from build123d import *

# Parameters (mm, degrees)
BOSS_EXTRUDE1_DEPTH      = 10.5
BOSS_EXTRUDE1_DEPTH_BACK = 10.5
SKETCH1_R                = 26.5
SKETCH1_R_2              = 7.5
BOSS_EXTRUDE2_DEPTH      = 8
BOSS_EXTRUDE2_DEPTH_BACK = 8
SKETCH3_R                = 7.5
SKETCH3_R_2              = 2.5


with BuildPart() as part:
    # Sketch1 → Boss-Extrude1 (new, two sides: drawn at the far end of the back side and taken through both)
    with BuildSketch(Plane.XY.offset(-BOSS_EXTRUDE1_DEPTH_BACK)):
        Circle(SKETCH1_R)
        Circle(SKETCH1_R_2, mode=Mode.SUBTRACT)
    extrude(amount=BOSS_EXTRUDE1_DEPTH + BOSS_EXTRUDE1_DEPTH_BACK)

    # Sketch3 → Boss-Extrude2 (add, two sides: drawn at the far end of the back side and taken through both)
    with BuildSketch(Plane.XY.offset(-BOSS_EXTRUDE2_DEPTH_BACK)):
        Circle(SKETCH3_R)
        Circle(SKETCH3_R_2, mode=Mode.SUBTRACT)
    extrude(amount=BOSS_EXTRUDE2_DEPTH + BOSS_EXTRUDE2_DEPTH_BACK)


solid = part.part
Here's how the part is built. I have some questions about the finished solid (model axes, mm). A direction names the side the tool comes from. Round coordinates to 2 decimals unless told otherwise and drop trailing zeros. Loops run counter-clockwise (first coordinate to the right, second up) from the corner with the lowest first, then second, coordinate; pieces in that order, holes last. Notation, with made-up numbers: M -12.75,-7.75 L 7.25,-7.75 A34 ccw 7.25,27.25 Z; hole C 11.25,63.25 d3. An arc over 180 degrees is marked long. Write each question's results on one line, items separated by ' | '. Start each with the question number.
(1) I want a section at C-C (z = -7.25). Please give me the cut outline in (x, y), then the cut area to 3 significant figures.
(2) I want a section at A-A (x = 0). Please give me the cut outline in (y, z).
(3) On a 3-axis mill with a long thin cutter (end or side, diameter ignored), from which of +Z, -Z, +X, -X, +Y, -Y can I reach the whole of each face in a straight line? I mean faces 1 (the flat face through (-2, 2, 8)), 2 (the flat face through (6, -6, -10.5)), 3 (the cylindrical face through (-7.493, 0.33, -9.268)). Say none if no direction works.
(4) I want a section at D-D (y = 12). Please give me the cut outline in (x, z), then the cut area to 3 significant figures.
(5) If I drill on probe 1 along Y at (x, z) = (0, 9.6); probe 2 along X at (y, z) = (-2, -1); probe 3 along Z at (x, y) = (-5.5, 2), over which ranges is the centre line in solid material (lowest first)? Write a range as from..to.
(6) Will these pins go through, and if not, where does the flat tip stop? P1, Ø4.5, axis at x = 3.5, y = 2.5, coming from the -Z side; P2, Ø5, axis at y = -7, z = -5.5, coming from the +X side; P3, Ø1.5, axis at x = -9.5, z = -5, coming from the -Y side.
(7) Thinking about a two-plate mould opening in X: for faces 4 (the cylindrical face through (14.246, 22.345, -0.147)), 5 (the flat face through (-2, 2, -8)), 6 (the flat face through (6, -6, 10.5)), which applies, pulls with the +X half, pulls with the -X half, needs draft (parallel to the pull), parting line crosses it, or undercut?
Solved:
1) outline: C 0,0 d53; hole C 0,0 d5 | area: 2,190 mm²
2) outline: M -26.5,-10.5 L -7.5,-10.5 L -7.5,-8 L -2.5,-8 L -2.5,8 L -7.5,8 L -7.5,10.5 L -26.5,10.5 Z; M 2.5,-8 L 7.5,-8 L 7.5,-10.5 L 26.5,-10.5 L 26.5,10.5 L 7.5,10.5 L 7.5,8 L 2.5,8 Z
3) face 1: +Z | face 2: -Z, +X, -X, +Y, -Y | face 3: -Z
4) outline: M -23.63,-10.5 L 23.63,-10.5 L 23.63,10.5 L -23.63,10.5 Z | area: 992 mm²
5) probe 1: y = -26.5..-7.5, 7.5..26.5 | probe 2: x = -26.42..-1.5, 1.5..26.42 | probe 3: z = -8..8
6) P1: stops at z = -8 | P2: stops at x = 26.12 | P3: stops at y = -25.01
7) face 4: parting line crosses it | face 5: undercut | face 6: needs draft
